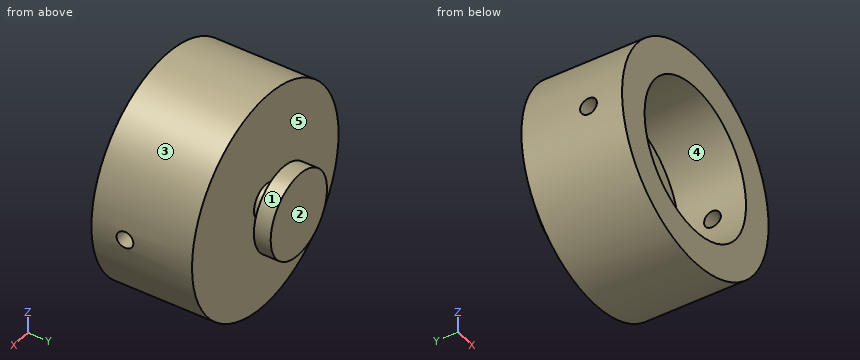
Solid Edge part; units mm, degrees
sketch "Sketch1" plane through (0, 0, 0) normal (0, -1, 0) x (1, 0, 0)
  circle A0 centre (0, 0) radius 6.5
extrude "Protrusion1" add sketch "Sketch1" against normal blind 6
sketch "Sketch2" plane through (0, 0, 0) normal (0, -1, 0) x (1, 0, 0)
  circle A0 centre (0, 0) radius 4.5
extrude "ExtrudedCutout_1" cut sketch "Sketch2" against normal blind 4
sketch "Sketch3" plane through (6.5, 3, 0) normal (1, 0, 0) x (0, -1, 0)
  circle A0 centre (1, 0) radius 0.5
extrude "ExtrudedCutout_2" cut sketch "Sketch3" against normal blind 17.8502
sketch "Sketch4" plane through (0, 6, 0) normal (0, 1, 0) x (1, 0, 0)
  circle A0 centre (0, 0) radius 1
extrude "ExtrudedProtrusion_2" add sketch "Sketch4" along normal blind 2
sketch "Sketch5" plane through (0, 8, 0) normal (0, 1, 0) x (1, 0, 0)
  circle A0 centre (0, 0) radius 2.5
extrude "ExtrudedProtrusion_3" add sketch "Sketch5" against normal blind 1
Could you check a few things on this model? Use its own coordinates, in mm. Face numbers are marked on the shaded views. A direction names the side the tool comes from. Give positions to 0.01 mm unless a question says otherwise; leave off trailing zeros. Loops run counter-clockwise (first coordinate to the right, second up) from the corner with the lowest first, then second, coordinate; pieces in that order, holes last. Notation, with made-up numbers: (11, -37.75) -> (62, -37.75) arc R13 ccw to (62, -19.75) -> close; hole circle Ø1 at (-16, 41). An arc over 180 degrees is marked (long way). Return JSON: item names as keys, results as strings.
Item 1: If we section it at B-B on z = 2: List the corners of the cut face in (x, y) for me.
Geometry results:
{"outline": "(-6.18, 0) -> (-4.03, 0) -> (-4.03, 4) -> (4.03, 4) -> (4.03, 0) -> (6.18, 0) -> (6.18, 6) -> (-6.18, 6) -> close; (-1.5, 7) -> (1.5, 7) -> (1.5, 8) -> (-1.5, 8) -> close"}
Item 2: If we section it at D-D on x = 0: List the corners of the cut face in (y, z) for me.
Geometry results:
{"outline": "(0, -6.5) -> (6, -6.5) -> (6, -1) -> (7, -1) -> (7, -2.5) -> (8, -2.5) -> (8, 2.5) -> (7, 2.5) -> (7, 1) -> (6, 1) -> (6, 6.5) -> (0, 6.5) -> (0, 4.5) -> (4, 4.5) -> (4, -4.5) -> (0, -4.5) -> close"}
Item 3: If we section it at A-A on z = 0: List the corners of the cut face in (x, y) for me, plus the area to 3 significant figures.
Geometry results:
{"outline": "(-6.5, 0) -> (-4.5, 0) -> (-4.5, 1.5) -> (-6.5, 1.5) -> close; (-6.5, 2.5) -> (-4.5, 2.5) -> (-4.5, 4) -> (4.5, 4) -> (4.5, 2.5) -> (6.5, 2.5) -> (6.5, 6) -> (1, 6) -> (1, 7) -> (2.5, 7) -> (2.5, 8) -> (-2.5, 8) -> (-2.5, 7) -> (-1, 7) -> (-1, 6) -> (-6.5, 6) -> close; (4.5, 0) -> (6.5, 0) -> (6.5, 1.5) -> (4.5, 1.5) -> close", "area": "45.0 mm²"}
Item 4: If we section it at C-C on y = 2: List the corners of the cut face in (x, z) for me.
Geometry results:
{"outline": "(-6.48, -0.5) arc R6.5 ccw to (6.48, -0.5) -> (4.47, -0.5) arc R4.5 cw to (-4.47, -0.5) -> close; (-6.48, 0.5) -> (-4.47, 0.5) arc R4.5 cw to (4.47, 0.5) -> (6.48, 0.5) arc R6.5 ccw to start"}
Item 5: We'd pull the mould along X, two halves only. Please class the marked faces 3, 4 and 5: +X half, -X half, draft (parallel to the pull), parting line (faces both ways), or undercut.
Geometry results:
{"face 3": "parting line", "face 4": "undercut", "face 5": "draft"}
Item 6: I'm going to push flat-ended pins straight in: pin 1 (4 mm diameter, centred on x = -0.5, z = 0, fed in from -Y); pin 2 (1.5 mm diameter, centred on x = 2, y = 2.5, fed in from -Z). Where does each tip first touch, or does it pass through?
Geometry results:
{"pin 1": "stops at y = 4", "pin 2": "stops at z = -6.38"}
Item 7: I need wall thicknesses on L1, parallel to X at y = 1.05, z = 0; L2, parallel to Y at x = -1.25, z = 1; L3, parallel to Y at x = 5.45, z = 0. Which ranges of each line are inside material? Lowest first, please. Write a range as from..to.
Geometry results:
{"L1": "x = -6.5..-4.5, 4.5..6.5", "L2": "y = 4..6, 7..8", "L3": "y = 0..1.5, 2.5..6"}
Item 8: Which directions (+Z, -Z, +X, -X, +Y, -Y) give clear straight access to the entire face, cutting with the end or side of a thin tool? Please do the marked faces 1 and 2.
Geometry results:
{"face 1": "+Y", "face 2": "+Z, -Z, +X, -X, +Y"}
